Autodesk Inventor part; units mm, degrees
ref_plane "YZ Plane" through (0, 0, 0) normal (1, 0, 0) x (0, 1, 0)
ref_plane "XZ Plane" through (0, 0, 0) normal (0, 1, 0) x (-1, 0, 0)
ref_plane "XY Plane" through (0, 0, 0) normal (0, 0, 1) x (1, 0, 0)
sketch "Boceto1" plane through (0, 0, 0) normal (0, 0, 1) x (1, 0, 0)
  circle A0 centre (0, 0) radius 9.525
  circle A1 centre (0, 0) radius 11.025
  dimension "d0" = 19.05
  dimension "d1" = 22.05
extrude "Extrusión1" add sketch "Boceto1" along normal mid plane 6.35
sketch "Boceto2" plane through (0, 0, 0) normal (1, 0, 0) x (0, 1, 0)
  line L0 (11.025, 3.175) -> (13.725, 3.175)
  line L1 (14.025, 3.475) -> (14.025, 4.375)
  line L2 (13.725, 4.675) -> (11.025, 4.675)
  arc A0 (11.025, 4.675) -> (9.525, 3.175) centre (11.025, 3.175) ccw
  arc A1 (13.725, 3.175) -> (14.025, 3.475) centre (13.725, 3.475) ccw
  arc A2 (14.025, 4.375) -> (13.725, 4.675) centre (13.725, 4.375) ccw
  line L3 (11.025, 3.175) -> (9.525, 3.175)
  line L4 (0, -0.9971) -> (0, 5.9828)
  point P0 (0, 0)
  point P1 (14.025, 3.175)
  point P2 (14.025, 4.675)
  dimension "d4" = 3
  dimension "d5" = 1.5
  dimension "d6" = 3
  dimension "d7" = 0.3
revolve "Revolución1" add sketch "Boceto2" angle 360 about axis through (0, 0, -10) along (0, 0, 1)
properties part number "Buje soporte superior"
Source: CAD feature listing. Evaluate the final solid. Frame: model axes, mm. A direction names the side the tool comes from. Coordinates: 2 decimals unless noted, no trailing zeros. Order: outer loops, then holes, each group sorted by start corner. A loop starts at its lowest first (then second) coordinate and runs counter-clockwise, first axis right, second up. Notation, with made-up numbers: (64, 84.5) - (94, 84.5) arc R10 ccw to (94, 103.5) - close; hole circle Ø1 at (50, 38.25). An arc over 180 degrees is marked (long way). One line per item, written item: value.
1) Mould query, pull axis X, two halves, no side actions, for faces 1 (the face through (-10, 0, -3.175)), 2 (the face through (-7.559, 5.796, -0.044)), 3 (the face through (-11.826, 7.54, 3.931)). Classes: released by +X, released by -X, zero draft, split by the parting line, or undercut.
Computed values:
face 1: zero draft
face 2: undercut
face 3: split by the parting line
2) Ray query, line 1 (X direction, y = 0, z = -1.5) (3 decimals); line 2 (X direction, y = 3.25, z = -1.5). Return the intervals inside material, ascending. Write a range as [from, to].
Computed values:
line 1: x = [-11.025, -9.525], [9.525, 11.025]
line 2: x = [-10.54, -8.95], [8.95, 10.54]
3) Cut plane C-C on z = 2.25. Output: boundary loops of the cut face in (x, y) (3 decimals).
Computed values:
outline: circle Ø22.05 at (0, 0); hole circle Ø19.05 at (0, 0)
4) Contact query for flat-ended pins moving along their axis: pin 1 (4 mm diameter, centred on y = 7.5, z = 2, fed in from +X); pin 2 (4 mm diameter, centred on x = 7, z = 3.5, fed in from +Y); pin 3 (4 mm diameter, centred on y = 5.5, z = 1, fed in from -X). Output: stop coordinate, or through.
Computed values:
pin 1: stops at x = 12.64
pin 2: stops at y = 13.1
pin 3: stops at x = -10.45
5) Reachability of faces 4 (the face through (-11.2, -0.1, 4.675)), 5 (the face through (-11.2, -0.1, 3.175)) from +Z, -Z, +X, -X, +Y, -Y: full face, straight path, thin tool, end or side. Return the list, or none.
Computed values:
face 4: +Z, +X, -X, +Y, -Y
face 5: -Z
6) Cut plane A-A on y = 0. Output: boundary loops of the cut face in (x, z) (3 decimals).
Computed values:
outline: (-14.025, 3.475) arc R0.3 ccw to (-13.725, 3.175) - (-11.025, 3.175) - (-11.025, -3.175) - (-9.525, -3.175) - (-9.525, 3.175) arc R1.5 ccw to (-11.025, 4.675) - (-13.725, 4.675) arc R0.3 ccw to (-14.025, 4.375) - close; (9.525, -3.175) - (11.025, -3.175) - (11.025, 3.175) - (13.725, 3.175) arc R0.3 ccw to (14.025, 3.475) - (14.025, 4.375) arc R0.3 ccw to (13.725, 4.675) - (11.025, 4.675) arc R1.5 ccw to (9.525, 3.175) - close
